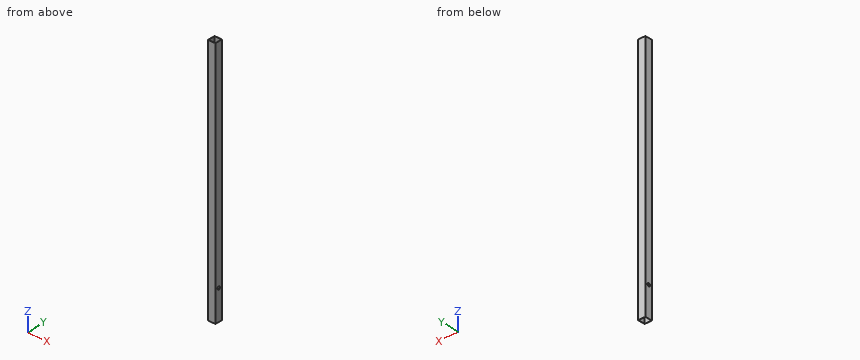
```python
from build123d import *

# Parameters (mm, degrees)
SKETCH1_W           = 20
SKETCH1_H           = 20
BOSS_EXTRUDE1_DEPTH = 660
SKETCH2_W           = 19
SKETCH2_H           = 19
CUT_EXTRUDE1_DEPTH  = 660
SKETCH3_R           = 4
CUT_EXTRUDE2_DEPTH  = 20


with BuildPart() as part:
    # Sketch1 → Boss-Extrude1 (new body)
    with BuildSketch(Plane.XY):
        Rectangle(SKETCH1_W, SKETCH1_H)
    extrude(amount=BOSS_EXTRUDE1_DEPTH)

    # Sketch2 → Cut-Extrude1 (cut)
    with BuildSketch(Plane(origin=(0, 0, 0), x_dir=(-1, 0, 0), z_dir=(0, 0, -1))):
        Rectangle(SKETCH2_W, SKETCH2_H)
    extrude(amount=-CUT_EXTRUDE1_DEPTH, mode=Mode.SUBTRACT)

    # Sketch3 → Cut-Extrude2 (cut)
    with BuildSketch(Plane(origin=(10, 0, 0), x_dir=(0, 0, -1), z_dir=(1, 0, 0))):
        with Locations(Location((-80, 0, 0), (0, 0, 90))):
            Circle(SKETCH3_R)
    extrude(amount=-CUT_EXTRUDE2_DEPTH, mode=Mode.SUBTRACT)


solid = part.part
```
For this review, take the finished solid that the model builds, in its own axes (mm). Round coordinates to 2 decimals unless told otherwise and drop trailing zeros. Order: outer loops, then holes, each group sorted by start corner. A loop starts at its lowest first (then second) coordinate and runs counter-clockwise, first axis right, second up.
Q1. We need section A-A, the plane y = 0. Give the boundary of the cut face in (x, z).
Findings below:
outline: (-10, 0) - (-9.5, 0) - (-9.5, 76) - (-10, 76) - close; (-10, 84) - (-9.5, 84) - (-9.5, 660) - (-10, 660) - close; (9.5, 0) - (10, 0) - (10, 76) - (9.5, 76) - close; (9.5, 84) - (10, 84) - (10, 660) - (9.5, 660) - close
Q2. We need section C-C, the plane x = -1.25. Give the boundary of the cut face in (y, z), plus the area to 3 significant figures.
Findings below:
outline: (-10, 0) - (-9.5, 0) - (-9.5, 660) - (-10, 660) - close; (9.5, 0) - (10, 0) - (10, 660) - (9.5, 660) - close
area: 660 mm2
Q3. Insertion check: P1, Ø2, axis at x = -5.5, y = -7, coming from the +Z side. The pin has a flat end and moves straight along its axis. Give the tip position at first contact, or say it passes through.
Findings below:
P1: passes through
Q4. We need section B-B, the plane z = 573.5. Give the boundary of the cut face in (x, y).
Findings below:
outline: (-10, -10) - (10, -10) - (10, 10) - (-10, 10) - close; hole (-9.5, -9.5) - (9.5, -9.5) - (9.5, 9.5) - (-9.5, 9.5) - close
Q5. Wall thickness on line 1 (Y direction, x = -1.5, z = 273.5); line 2 (Z direction, x = -9.55, y = 0): over which ranges is each line inside the solid? List them lowest first.
Findings below:
line 1: y = -10 to -9.5, 9.5 to 10
line 2: z = 0 to 76, 84 to 660
